Can you work these out from the model? Positions are in its coordinate system, mm. A direction names the side the tool comes from. Round coordinates to 2 decimals unless told otherwise and drop trailing zeros. Loops run counter-clockwise (first coordinate to the right, second up) from the corner with the lowest first, then second, coordinate; pieces in that order, holes last.
from build123d import *

# Parameters (mm, degrees)
SKETCH2_W           = 60
SKETCH2_H           = 100
BOSS_EXTRUDE1_DEPTH = 10
SKETCH1_W           = 6.35
SKETCH1_H           = 18
CUT_EXTRUDE1_DEPTH  = 10


with BuildPart() as part:
    # Sketch2 → Boss-Extrude1 (new body)
    with BuildSketch(Plane(origin=(0, 0, 0), x_dir=(1, 0, 0), z_dir=(0, 1, 0))):
        with Locations((30, 50)):
            Rectangle(SKETCH2_W, SKETCH2_H)
    extrude(amount=BOSS_EXTRUDE1_DEPTH)

    # Sketch1 → Cut-Extrude1 (cut)
    with BuildSketch(Plane(origin=(0, 0, 0), x_dir=(1, 0, 0), z_dir=(0, 1, 0))):
        with Locations((8.175, 14)):
            Rectangle(SKETCH1_W, SKETCH1_H)
        with Locations((8.175, 50)):
            Rectangle(SKETCH1_W, SKETCH1_H)
        with Locations((8.175, 86)):
            Rectangle(SKETCH1_W, SKETCH1_H)
        with Locations((51.825, 86)):
            Rectangle(SKETCH1_W, SKETCH1_H)
        with Locations((51.825, 50)):
            Rectangle(SKETCH1_W, SKETCH1_H)
        with Locations((51.825, 14)):
            Rectangle(SKETCH1_W, SKETCH1_H)
    extrude(amount=CUT_EXTRUDE1_DEPTH, mode=Mode.SUBTRACT)


solid = part.part
(1) If we section it at C-C, the plane y = 4: List the corners of the cut face in (x, z) for me.
Worked answers:
outline: (0, -100) - (60, -100) - (60, 0) - (0, 0) - close; hole (5, -95) - (11.35, -95) - (11.35, -77) - (5, -77) - close; hole (5, -59) - (11.35, -59) - (11.35, -41) - (5, -41) - close; hole (5, -23) - (11.35, -23) - (11.35, -5) - (5, -5) - close; hole (48.65, -95) - (55, -95) - (55, -77) - (48.65, -77) - close; hole (48.65, -59) - (55, -59) - (55, -41) - (48.65, -41) - close; hole (48.65, -23) - (55, -23) - (55, -5) - (48.65, -5) - close
(2) For faces 3 (the flat face through (8, 5, -23)), 4 (the flat face through (60, 5, -49)), which set-ups out of +Z, -Z, +X, -X, +Y, -Y let a thin tool reach every point of the face, with its end or its side?
Worked answers:
face 3: +Y, -Y
face 4: +Z, -Z, +X, +Y, -Y
(3) If we mould it in two halves opening along Z, with no side actions, what happens to faces 1 (the flat face through (52, 5, -59)), 2 (the flat face through (30, 10, -51))? For each: released by +Z, released by -Z, zero draft, split by the parting line, or undercut.
Worked answers:
face 1: undercut
face 2: zero draft
(4) If we section it at B-B, the plane x = 53: List the corners of the cut face in (y, z) for me.
Worked answers:
outline: (0, -100) - (10, -100) - (10, -95) - (0, -95) - close; (0, -77) - (10, -77) - (10, -59) - (0, -59) - close; (0, -41) - (10, -41) - (10, -23) - (0, -23) - close; (0, -5) - (10, -5) - (10, 0) - (0, 0) - close
(5) If we section it at A-A, the plane z = -81.5: List the corners of the cut face in (x, y) for me, then the cut area to 3 significant figures.
Worked answers:
outline: (0, 0) - (5, 0) - (5, 10) - (0, 10) - close; (11.35, 0) - (48.65, 0) - (48.65, 10) - (11.35, 10) - close; (55, 0) - (60, 0) - (60, 10) - (55, 10) - close
area: 473 mm2
(6) If I drill on line 1 (Z direction, x = 9, y = 8); line 2 (X direction, y = 9, z = -84), over which ranges is the centre line in solid material (lowest first)?
Worked answers:
line 1: z = -100 to -95, -77 to -59, -41 to -23, -5 to 0
line 2: x = 0 to 5, 11.35 to 48.65, 55 to 60
